Verification items for this drawing (mm, ordinates from the low corner). A direction names the side the tool comes from. Coordinates: 2 decimals unless noted, no trailing zeros. Order: outer loops, then holes, each group sorted by start corner. A loop starts at its lowest first (then second) coordinate and runs counter-clockwise, first axis right, second up. Notation, with made-up numbers: M 58,58 L 77,58 A30 ccw 77,95 Z; hole C 33.25,76.5 d10. An arc over 180 degrees is marked long. Answer as a JSON object with one key per item and string values. Group by question number.
(1) Cross-section at A-A (x = 42.5). Enter the section's corners in (y, z).
(2) Cross-section at B-B (z = 6.5). Enter the section's corners in (x, y) (1 decimal).
(3) Material ranges on line 1 (Z direction, x = 49.5, y = 3.75); line 2 (X direction, y = 3, z = 15) (1 decimal); line 3 (Z direction, x = 150.5, y = 4.75) (1 decimal), recorded low to high.
(4) Gauge pin test, flat ends, axial feed: pin 1 Ø1 at (y, z) = (4, 23.5) entering from -X; pin 2 Ø1 at (y, z) = (2.5, 38.5) entering from -X (1 decimal); pin 3 Ø1.5 at (y, z) = (7, 18) entering from +X. Record the tip position at first contact, or that the pin passes through.
(5) Access from +Z, -Z, +X, -X, +Y, -Y to the whole of each face (thin tool, end or side, straight path). Record for the marked faces 4 and 5.
(6) Mould release check, pull along Z, two halves, no side actions. Record for the marked faces 1, 2 and 3: released by +Z, released by -Z, zero draft, split by the parting line, or undercut.
(7) Cross-section at C-C (y = 6.5). Enter the section's corners in (x, z).
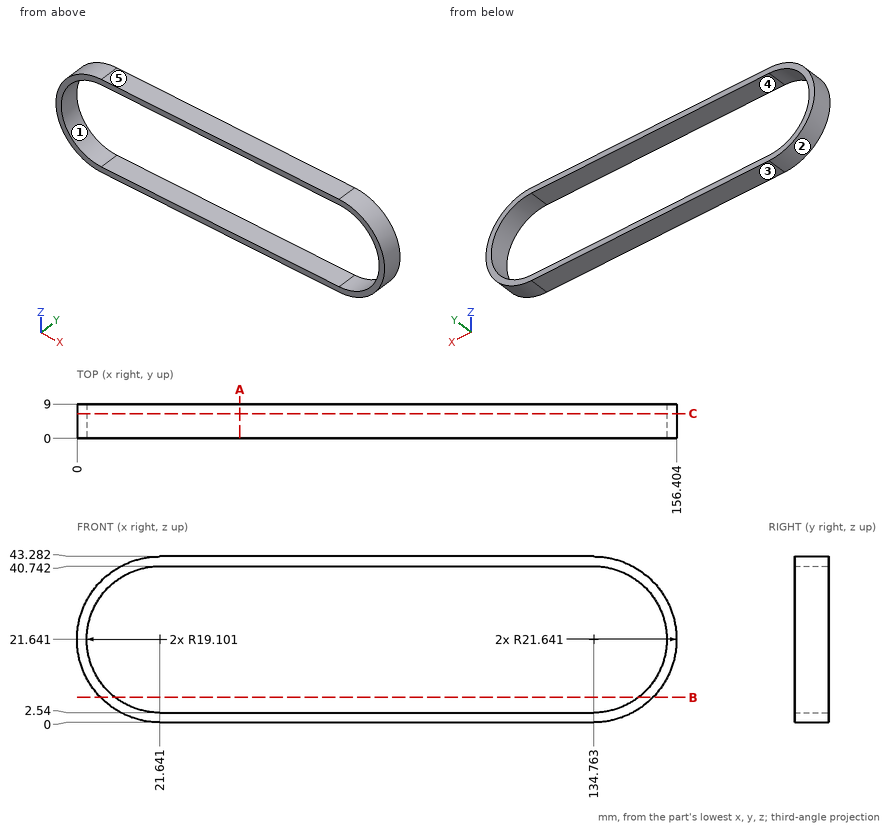
Taken from the geometry:
{
 "1": {"outline": "M 0,0 L 9,0 L 9,2.54 L 0,2.54 Z; M 0,40.74 L 9,40.74 L 9,43.28 L 0,43.28 Z"},
 "2": {"outline": "M 6.2,0 L 10,0 L 10,9 L 6.2,9 Z; M 146.4,0 L 150.2,0 L 150.2,9 L 146.4,9 Z"},
 "3": {"line 1": "z = 0 to 2.54, 40.74 to 43.28", "line 2": "x = 1 to 3.7, 152.7 to 155.4", "line 3": "z = 6.8 to 10.8, 32.5 to 36.5"},
 "4": {"pin 1": "stops at x = 0.04", "pin 2": "stops at x = 7.5", "pin 3": "stops at x = 156.21"},
 "5": {"face 4": "+Y, -Y", "face 5": "+Z, +X, -X, +Y, -Y"},
 "6": {"face 1": "undercut", "face 2": "split by the parting line", "face 3": "released by -Z"},
 "7": {"outline": "M 21.64,0 L 134.76,0 A21.64 ccw 134.76,43.28 L 21.64,43.28 A21.64 ccw Z; hole M 21.64,2.54 L 134.76,2.54 A19.1 ccw 134.76,40.74 L 21.64,40.74 A19.1 ccw Z"}
}
